Geometry: final body of the model. Coordinates: model frame, mm. A direction names the side the tool comes from. Coordinates: 2 decimals unless noted, no trailing zeros. Write each loop counter-clockwise with the first axis right and the second up, starting at its lowest first coordinate (ties: lowest second). Pieces come first, ordered by that corner, then holes. Notation, with made-up numbers: (71.25, 56.25) - (123.25, 56.25) arc R28 cw to (123.25, 75.25) - close; hole circle Ø7 at (-9, 78.5). An arc over 180 degrees is marked (long way). Put each result on its own line as item: value.
```python
from build123d import *

# Parameters (mm, degrees)
BOSS_EXTRUDE1_OUTLINE_R  = 0.7
BOSS_EXTRUDE1_DEPTH      = 2
BOSS_EXTRUDE2_DEPTH      = 0.86
BOSS_EXTRUDE2_DEPTH_BACK = 1
SKETCH2_W                = 15.014867696
SKETCH2_H                = 2
SKETCH3_W                = 8
SKETCH3_H                = 5
CUT_EXTRUDE1_DEPTH       = 23.82865975
SKETCH4_W                = 15.014867696
SKETCH4_H                = 1.5
BOSS_EXTRUDE3_DEPTH      = 5
SKETCH5_W                = 8
SKETCH5_H                = 4
CUT_EXTRUDE2_DEPTH       = 3
BOSS_EXTRUDE5_DEPTH      = 20
SKETCH9_R                = 1.275
CUT_EXTRUDE3_DEPTH       = 0.8
HOLE1_START              = -3
HOLE1_OUTLINE_R          = 1.25
HOLE1_DEPTH              = 5
HOLE2_START              = -3
HOLE2_DEPTH              = 5


# Read off the part's stored shape, not the designer's step: Boss-Extrude1, Hole1, Hole2
with BuildPart() as part:
    # Boss-Extrude1 outline → Boss-Extrude1 (new body)
    with BuildSketch(Plane.XY):
        with BuildLine():
            ThreePointArc((7.514083588, 19.508491868), (7.257921972, 20.275277178), (6.518471313, 20.602066422))
            Line((6.518471313, 20.602066422), (-6.496396384, 20.602066422))
            ThreePointArc((-6.496396384, 20.602066422), (-7.234510066, 20.276742783), (-7.49237209, 19.512442807))
            Line((-7.49237209, 19.512442807), (-5.630745451, -1.175574425))
            ThreePointArc((-5.630745451, -1.175574425), (-5.309446106, -1.824064491), (-4.634769745, -2.085950809))
            Line((-4.634769745, -2.085950809), (4.574067822, -2.085950809))
            ThreePointArc((4.574067822, -2.085950809), (5.247278579, -1.825401468), (5.569680097, -1.179525363))
            Line((5.569680097, -1.179525363), (7.514083588, 19.508491868))
        make_face()
        Circle(BOSS_EXTRUDE1_OUTLINE_R, mode=Mode.SUBTRACT)
        with Locations((-5.999999992, 17.596194699)):
            Circle(BOSS_EXTRUDE1_OUTLINE_R, mode=Mode.SUBTRACT)
        with Locations((6.000000016, 17.596194697)):
            Circle(BOSS_EXTRUDE1_OUTLINE_R, mode=Mode.SUBTRACT)
    extrude(amount=BOSS_EXTRUDE1_DEPTH)

    # Sketch2 → Boss-Extrude2 (add, two sides: drawn at the far end of the back side and taken through both)
    with BuildSketch(Plane(origin=(0, 20.602066422, 0), x_dir=(1, 0, 0), z_dir=(0, 1, 0)).offset(-BOSS_EXTRUDE2_DEPTH_BACK)):
        with Locations((0.011037464, -1)):
            Rectangle(SKETCH2_W, SKETCH2_H)
    extrude(amount=BOSS_EXTRUDE2_DEPTH + BOSS_EXTRUDE2_DEPTH_BACK)

    # Sketch3 → Cut-Extrude1 (cut, through all)
    with BuildSketch(Plane(origin=(0, 0, 0), x_dir=(-1, 0, 0), z_dir=(0, 0, -1))):
        with Locations((-0.011037464, 21.462066422)):
            Rectangle(SKETCH3_W, SKETCH3_H)
    extrude(amount=-CUT_EXTRUDE1_DEPTH, mode=Mode.SUBTRACT)

    # Sketch4 → Boss-Extrude3 (add)
    with BuildSketch(Plane.XY.offset(2)):
        with Locations((0.011037464, 22.212066422)):
            Rectangle(SKETCH4_W, SKETCH4_H)
    extrude(amount=-BOSS_EXTRUDE3_DEPTH)

    # Sketch5 → Cut-Extrude2 (cut)
    with BuildSketch(Plane(origin=(0, 22.962066422, 0), x_dir=(1, 0, 0), z_dir=(0, 1, 0))):
        with Locations((0.011037464, -2)):
            Rectangle(SKETCH5_W, SKETCH5_H)
    extrude(amount=-CUT_EXTRUDE2_DEPTH, mode=Mode.SUBTRACT)

    # Sketch6 → Boss-Extrude5 (add)
    with BuildSketch(Plane(origin=(0, 22.962066422, 0), x_dir=(1, 0, 0), z_dir=(0, 1, 0))):
        Polygon((-3.988962536, 0), (4.011037464, 0), (4.011037464, -2), (7.518471312, -2), (7.518471312, 3), (-7.496396384, 3), (-7.496396384, -2), (-3.988962536, -2), align=None)
    extrude(amount=BOSS_EXTRUDE5_DEPTH)

    # Sketch9 → Cut-Extrude3 (cut)
    with BuildSketch(Plane.XY.offset(2)):
        with Locations((-5.999999992, 17.596194699)):
            Circle(SKETCH9_R)
        with Locations((6.000000016, 17.596194697)):
            Circle(SKETCH9_R)
        Circle(SKETCH9_R)
    extrude(amount=-CUT_EXTRUDE3_DEPTH, mode=Mode.SUBTRACT)

    # Hole1 outline → Hole1 (cut)
    with BuildSketch(Plane.XY.offset(HOLE1_START)):
        with Locations((-5.881528688, 40.468009485)):
            Circle(HOLE1_OUTLINE_R)
        with Locations((5.718471312, 40.468009485)):
            Circle(HOLE1_OUTLINE_R)
    extrude(amount=HOLE1_DEPTH, mode=Mode.SUBTRACT)

    # Hole2 outline → Hole2 (cut)
    with BuildSketch(Plane.XY.offset(HOLE2_START)):
        with BuildLine():
            ThreePointArc((5.811037464, 41.714577376), (6.968471312, 40.468009485), (5.811037464, 39.221441594))
            ThreePointArc((5.811037464, 39.221441594), (7.153603616, 40.468009485), (5.811037464, 41.714577376))
        make_face()
        with BuildLine():
            ThreePointArc((-5.788962536, 41.714577376), (-4.631528688, 40.468009485), (-5.788962536, 39.221441594))
            ThreePointArc((-5.788962536, 39.221441594), (-4.446396384, 40.468009485), (-5.788962536, 41.714577376))
        make_face()
    extrude(amount=HOLE2_DEPTH, mode=Mode.SUBTRACT)


solid = part.part
```
1. Ray query, probe 1 along X at (y, z) = (37, 0.25); probe 2 along Y at (x, z) = (4, -1.95); probe 3 along Y at (x, z) = (0, 1.8) (3 decimals). Return the intervals inside material, ascending. Write a range as from..to.
Answer below:
probe 1: x = -7.5..-3.99, 4.01..7.52
probe 2: y = 21.46..42.96
probe 3: y = -2.086..-1.275, 1.275..18.962
2. Section query B-B (x = 0). Return loops of the section in (y, z) (3 decimals).
Answer below:
outline: (-2.086, 0) - (-0.7, 0) - (-0.7, 1.2) - (-1.275, 1.2) - (-1.275, 2) - (-2.086, 2) - close; (0.7, 0) - (18.962, 0) - (18.962, 2) - (1.275, 2) - (1.275, 1.2) - (0.7, 1.2) - close; (21.462, -3) - (42.962, -3) - (42.962, 0) - (21.462, 0) - close
3. Section query A-A (x = -2.25). Return loops of the section in (y, z).
Answer below:
outline: (-2.09, 0) - (18.96, 0) - (18.96, 2) - (-2.09, 2) - close; (21.46, -3) - (42.96, -3) - (42.96, 0) - (21.46, 0) - close
4. Section query D-D (y = 0). Return loops of the section in (x, z) (3 decimals).
Answer below:
outline: (-5.737, 0) - (-0.7, 0) - (-0.7, 1.2) - (-1.275, 1.2) - (-1.275, 2) - (-5.737, 2) - close; (0.7, 0) - (5.681, 0) - (5.681, 2) - (1.275, 2) - (1.275, 1.2) - (0.7, 1.2) - close
5. Section query C-C (y = 34). Return loops of the section in (x, z), then the cut area to 3 significant figures.
Answer below:
outline: (-7.5, -3) - (7.52, -3) - (7.52, 2) - (4.01, 2) - (4.01, 0) - (-3.99, 0) - (-3.99, 2) - (-7.5, 2) - close
area: 59.1 mm²
6. Mould query, pull axis Y, two halves, no side actions, for faces 1 (the flat face through (0, -2.086, 1)), 2 (the flat face through (0, 42.962, -1)), 3 (the cylindrical face through (-4.447, 40.439, -0.535)). Classes: +Y half, -Y half, draft (parallel to the pull), parting line (faces both ways), or undercut.
Answer below:
face 1: -Y half
face 2: +Y half
face 3: undercut
7. Pin query (flat end, axial travel): pin 1 Ø2 at (x, y) = (-6, 17.6) entering from -Z; pin 2 Ø4 at (x, y) = (-6, 17.6) entering from +Z; pin 3 Ø1.5 at (x, z) = (3.5, -2) entering from -Y; pin 4 Ø1.6 at (x, y) = (6, 17.6) entering from +Z. Return the tip coordinate at first contact, or that it passes through.
Answer below:
pin 1: stops at z = 0
pin 2: stops at z = 2
pin 3: stops at y = 21.46
pin 4: stops at z = 1.2
8. Set-up query: faces 4 (the flat face through (0, 10, 0)), 5 (the cylindrical face through (4.47, 40.5, -0.54)), 6 (the cylindrical face through (-5.317, -1.817, 0.986)), 7 (the cylindrical face through (-6.17, 18.86, 1.61)), 8 (the flat face through (-3.989, 31, 1)). Return all of +Z, -Z, +X, -X, +Y, -Y with unobstructed straight access to the full face (end or side cutting, diameter ignored); none if empty.
Answer below:
face 4: -Z, +X, -X, -Y
face 5: +Z, -Z
face 6: +Z, -Z, -X, -Y
face 7: +Z
face 8: +Z, +Y
